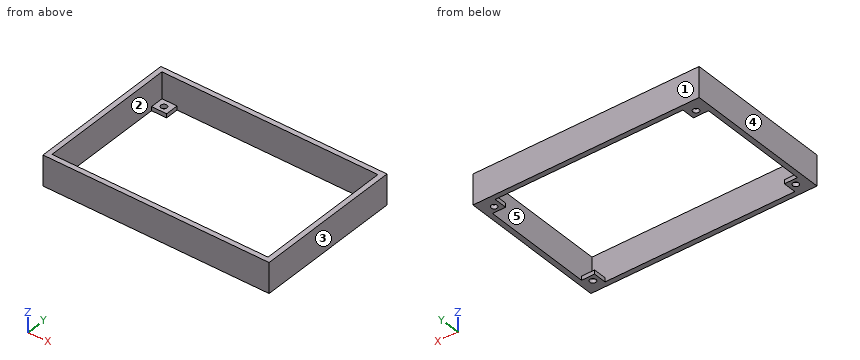
```python
from build123d import *

# Parameters (mm, degrees)
SKETCH_W      = 112
SKETCH_H      = 73.4
SKETCH_W_2    = 107
SKETCH_H_2    = 68.4
PAD_DEPTH     = 15
SKETCH001_W   = 6.5
SKETCH001_H   = 6.5
SKETCH001_W_2 = 7.5
PAD001_DEPTH  = 2
SKETCH002_R   = 1.5
POCKET_DEPTH  = 2


with BuildPart() as part:
    # Sketch → Pad (new body)
    with BuildSketch(Plane.XY):
        Rectangle(SKETCH_W, SKETCH_H)
        Rectangle(SKETCH_W_2, SKETCH_H_2, mode=Mode.SUBTRACT)
    extrude(amount=PAD_DEPTH)

    # Sketch001 (on Face9 of Pad) → Pad001 (join)
    with BuildSketch(Plane(origin=(0, 0, 0), x_dir=(1, 0, 0), z_dir=(0, 0, -1))):
        with Locations((-50.25, 30.95)):
            Rectangle(SKETCH001_W, SKETCH001_H)
        with Locations((-49.75, -30.95)):
            Rectangle(SKETCH001_W_2, SKETCH001_H)
        with Locations((50.25, 30.95)):
            Rectangle(SKETCH001_W, SKETCH001_H)
        with Locations((50.25, -30.95)):
            Rectangle(SKETCH001_W, SKETCH001_H)
    extrude(amount=-PAD001_DEPTH)

    # Sketch002 (on Face22 of Pad001) → Pocket (cut)
    with BuildSketch(Plane(origin=(0, 0, 0), x_dir=(1, 0, 0), z_dir=(0, 0, -1))):
        with Locations((-50.25, 30.75)):
            Circle(SKETCH002_R)
        with Locations((50.25, -30.75)):
            Circle(SKETCH002_R)
        with Locations((-49.75, -30.75)):
            Circle(SKETCH002_R)
        with Locations((50.25, 30.75)):
            Circle(SKETCH002_R)
    extrude(amount=-POCKET_DEPTH, mode=Mode.SUBTRACT)


solid = part.part
```
The model under review builds one solid part; all positions refer to its coordinate system, in mm. Face numbers are marked on the shaded views. A direction names the side the tool comes from. Give positions to 0.01 mm unless a question says otherwise; leave off trailing zeros. Write each loop counter-clockwise with the first axis right and the second up, starting at its lowest first coordinate (ties: lowest second). Pieces come first, ordered by that corner, then holes. Notation, with made-up numbers: (51, 17.25) -> (55, 17.25) arc R17 ccw to (55, 23.25) -> close; hole circle Ø7 at (-24.5, 3.5). An arc over 180 degrees is marked (long way). Answer in a Markdown table with one row per item.
1) Add section D-D on y = -13.5. State the section outline as (x, z) points.
Worked answers:
| item | result |
|---|---|
| outline | (-56, 0) -> (-53.5, 0) -> (-53.5, 15) -> (-56, 15) -> close; (53.5, 0) -> (56, 0) -> (56, 15) -> (53.5, 15) -> close |
2) Add section B-B on z = 3.5. State the section outline as (x, y) points.
Worked answers:
| item | result |
|---|---|
| outline | (-56, -36.7) -> (56, -36.7) -> (56, 36.7) -> (-56, 36.7) -> close; hole (-53.5, -34.2) -> (53.5, -34.2) -> (53.5, 34.2) -> (-53.5, 34.2) -> close |
3) Tool access review of the marked faces 1 and 2: name each direction out of +Z, -Z, +X, -X, +Y, -Y from which nothing blocks a thin tool from reaching the whole face with its end or side.
Worked answers:
| item | result |
|---|---|
| face 1 | +Z, -Z, +X, -X, +Y |
| face 2 | +Z |
4) Add section C-C on x = 50.25. State the section outline as (y, z) points.
Worked answers:
| item | result |
|---|---|
| outline | (-36.7, 0) -> (-32.25, 0) -> (-32.25, 2) -> (-34.2, 2) -> (-34.2, 15) -> (-36.7, 15) -> close; (-29.25, 0) -> (-27.7, 0) -> (-27.7, 2) -> (-29.25, 2) -> close; (27.7, 0) -> (29.25, 0) -> (29.25, 2) -> (27.7, 2) -> close; (32.25, 0) -> (36.7, 0) -> (36.7, 15) -> (34.2, 15) -> (34.2, 2) -> (32.25, 2) -> close |
5) Add section A-A on y = -30.75. State the section outline as (x, z) points, plus the area to 3 significant figures.
Worked answers:
| item | result |
|---|---|
| outline | (-56, 0) -> (-51.75, 0) -> (-51.75, 2) -> (-53.5, 2) -> (-53.5, 15) -> (-56, 15) -> close; (-48.75, 0) -> (-47, 0) -> (-47, 2) -> (-48.75, 2) -> close; (47, 0) -> (48.75, 0) -> (48.75, 2) -> (47, 2) -> close; (51.75, 0) -> (56, 0) -> (56, 15) -> (53.5, 15) -> (53.5, 2) -> (51.75, 2) -> close |
| area | 89.0 mm² |
6) Mouldability with a two-part tool opening along X and no side actions: class the marked faces 3, 4 and 5 as +X half, -X half, draft (parallel to the pull), parting line (faces both ways), or undercut.
Worked answers:
| item | result |
|---|---|
| face 3 | +X half |
| face 4 | -X half |
| face 5 | undercut |
7) Clearance check with flat-ended pins moving along their axes: P1, Ø2, axis at x = 49.5, y = -32.5, coming from the +Z side; P2, Ø4, axis at x = -50.25, y = -30.75, coming from the -Z side. State where each tip first meets the part, or that it passes through.
Worked answers:
| item | result |
|---|---|
| P1 | z = 2 |
| P2 | z = 0 |
8) For L1, parallel to Y at x = 50.25, z = 1; L2, parallel to X at y = 30.75, z = 0.65; L3, parallel to X at y = -30.5, z = 1.5, list the stretches that pass through material, from the lowest coordinate up. Write a range as [from, to].
Worked answers:
| item | result |
|---|---|
| L1 | [-36.7, -32.25], [-29.25, -27.7], [27.7, 29.25], [32.25, 36.7] |
| L2 | [-56, -51.25], [-48.25, -46], [47, 48.75], [51.75, 56] |
| L3 | [-56, -51.73], [-48.77, -47], [47, 48.77], [51.73, 56] |
